Work out the finished part from the listing and answer in its coordinate system (mm). Face numbers are marked on the shaded views. A direction names the side the tool comes from. Coordinates: 2 decimals unless noted, no trailing zeros. Loops run counter-clockwise (first coordinate to the right, second up) from the corner with the lowest first, then second, coordinate; pieces in that order, holes last. Notation, with made-up numbers: (56.25, 48) -> (85.25, 48) arc R10 ccw to (85.25, 55) -> close; hole circle Ø8 at (-4, -38). An arc over 180 degrees is marked (long way). Answer as CSV lines item,"result".
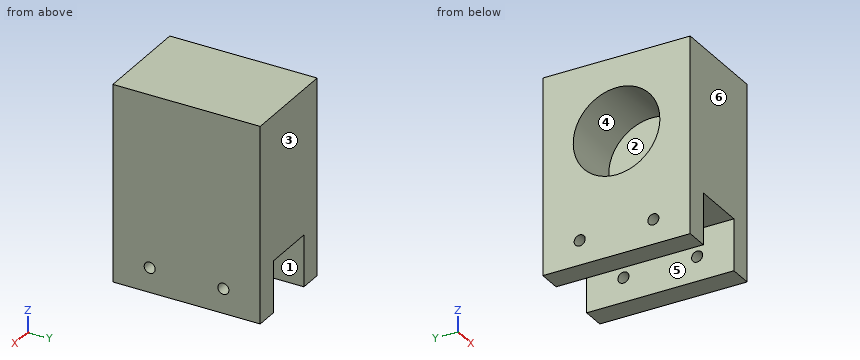
```python
from build123d import *

# Parameters (mm, degrees)
SKETCH1_W           = 60
SKETCH1_H           = 60
SKETCH1_R           = 17.65
BOSS_EXTRUDE1_DEPTH = 40
SKETCH4_W           = 10
SKETCH4_H           = 60
BOSS_EXTRUDE2_DEPTH = 20
SKETCH5_R           = 2.25
CUT_EXTRUDE1_DEPTH  = 71.710678119
BOSS_EXTRUDE3_START = -15
SKETCH6_R           = 17.65
BOSS_EXTRUDE3_DEPTH = 15
SKETCH7_W           = 21.5
SKETCH7_H           = 21
CUT_EXTRUDE2_DEPTH  = 88.749643874


with BuildPart() as part:
    # Sketch1 → Boss-Extrude1 (new body)
    with BuildSketch(Plane(origin=(0, 0, 0), x_dir=(0, 0, -1), z_dir=(1, 0, 0))):
        Rectangle(SKETCH1_W, SKETCH1_H)
        Circle(SKETCH1_R, mode=Mode.SUBTRACT)
    extrude(amount=BOSS_EXTRUDE1_DEPTH)

    # Sketch4 → Boss-Extrude2 (add)
    with BuildSketch(Plane(origin=(0, 0, -30), x_dir=(-1, 0, 0), z_dir=(0, 0, -1))):
        with Locations((-35, 0)):
            Rectangle(SKETCH4_W, SKETCH4_H)
    boss_extrude2 = extrude(amount=BOSS_EXTRUDE2_DEPTH)

    # Sketch5 → Cut-Extrude1 (cut, through all)
    with BuildSketch(Plane(origin=(40, 0, 0), x_dir=(0, 0, -1), z_dir=(1, 0, 0))):
        with Locations((40, -15)):
            Circle(SKETCH5_R)
        with Locations(Location((40, 15, 0), (0, 0, 90))):
            Circle(SKETCH5_R)
    cut_extrude1 = extrude(amount=-CUT_EXTRUDE1_DEPTH, mode=Mode.SUBTRACT)

    # Mirror1: Boss-Extrude2, Cut-Extrude1 across plane
    add(boss_extrude2.mirror(Plane(origin=(20, 0, 0), x_dir=(0, 0, 1), z_dir=(1, 0, 0))))
    add(cut_extrude1.mirror(Plane(origin=(20, 0, 0), x_dir=(0, 0, 1), z_dir=(1, 0, 0))), mode=Mode.SUBTRACT)

    # Sketch6 → Boss-Extrude3 (add)
    with BuildSketch(Plane(origin=(40, 0, 0), x_dir=(0, 0, -1), z_dir=(1, 0, 0)).offset(BOSS_EXTRUDE3_START)):
        Circle(SKETCH6_R)
    extrude(amount=BOSS_EXTRUDE3_DEPTH)

    # Sketch7 → Cut-Extrude2 (cut, through all)
    with BuildSketch(Plane(origin=(0, 30, 0), x_dir=(1, 0, 0), z_dir=(0, 1, 0))):
        with Locations((20, 39.5)):
            Rectangle(SKETCH7_W, SKETCH7_H)
    extrude(amount=-CUT_EXTRUDE2_DEPTH, mode=Mode.SUBTRACT)


solid = part.part
```
(1) A cutting plane is placed at C-C, the plane x = 14. Write down the section's boundary in (y, z), and give its area (3 significant figures).
Computed values:
outline,"(-30, -29) -> (30, -29) -> (30, 30) -> (-30, 30) -> close; hole circle Ø35.3 at (0, 0)"
area,"2,560 mm2"
(2) Flat-ended cylindrical pins translate along their axes: pin 1 Ø17.5 at (y, z) = (3.5, 0.5) entering from -X; pin 2 Ø6.5 at (x, y) = (16, -14) entering from -Z; pin 3 Ø3.5 at (y, z) = (-15, -40) entering from +X. Find the tip coordinate at first contact, or state that the pin passes through.
Computed values:
pin 1,"x = 25"
pin 2,"z = -29"
pin 3,"through"
(3) For a pull along X with two mould halves and no side action, classify the marked faces 1, 2 and 3 as pulls with the +X half, pulls with the -X half, needs draft (parallel to the pull), parting line crosses it, or undercut.
Computed values:
face 1,"undercut"
face 2,"pulls with the -X half"
face 3,"needs draft"
(4) A cutting plane is placed at A-A, the plane z = -40. Write down the section's boundary in (x, y).
Computed values:
outline,"(0, -30) -> (9.25, -30) -> (9.25, -17.25) -> (0, -17.25) -> close; (0, -12.75) -> (9.25, -12.75) -> (9.25, 12.75) -> (0, 12.75) -> close; (0, 17.25) -> (9.25, 17.25) -> (9.25, 30) -> (0, 30) -> close; (30.75, -30) -> (40, -30) -> (40, -17.25) -> (30.75, -17.25) -> close; (30.75, -12.75) -> (40, -12.75) -> (40, 12.75) -> (30.75, 12.75) -> close; (30.75, 17.25) -> (40, 17.25) -> (40, 30) -> (30.75, 30) -> close"
(5) A cutting plane is placed at B-B, the plane x = 3. Write down the section's boundary in (y, z), and give its area (3 significant figures).
Computed values:
outline,"(-30, -50) -> (30, -50) -> (30, 30) -> (-30, 30) -> close; hole circle Ø35.3 at (0, 0); hole circle Ø4.5 at (-15, -40); hole circle Ø4.5 at (15, -40)"
area,"3,790 mm2"
(6) Consider line 1 along X through (y, z) = (-17, -30); line 2 along Y through (x, z) = (5, -40); line 3 along Y through (x, z) = (16.25, 0). Determine where each line is inside the solid, lowest interval first.
Computed values:
line 1,"0 to 9.25, 30.75 to 40"
line 2,"-30 to -17.25, -12.75 to 12.75, 17.25 to 30"
line 3,"-30 to -17.65, 17.65 to 30"
(7) Which of the six approach directions +Z, -Z, +X, -X, +Y, -Y give full straight-line access (tool end or side, diameter ignored) to the marked faces 4, 5 and 6?
Computed values:
face 4,"-X"
face 5,"-Z, +Y, -Y"
face 6,"+Z, -Z, +X, -X, -Y"
(8) A cutting plane is placed at D-D, the plane y = -7.5. Write down the section's boundary in (x, z), and give its area (3 significant figures).
Computed values:
outline,"(0, -50) -> (9.25, -50) -> (9.25, -29) -> (30.75, -29) -> (30.75, -50) -> (40, -50) -> (40, 30) -> (0, 30) -> (0, 15.98) -> (25, 15.98) -> (25, -15.98) -> (0, -15.98) -> close"
area,"1,950 mm2"
